Autodesk Inventor part; units mm, degrees
ref_plane "YZ Plane" through (0, 0, 0) normal (1, 0, 0) x (0, 1, 0)
ref_plane "XZ Plane" through (0, 0, 0) normal (0, 1, 0) x (-1, 0, 0)
ref_plane "XY Plane" through (0, 0, 0) normal (0, 0, 1) x (1, 0, 0)
sketch "Sketch1" plane through (0, 0, 0) normal (0, 0, 1) x (1, 0, 0)
  line L0 (-25.4, -38.1) -> (25.4, -38.1) construction
  line L1 (25.4, -38.1) -> (25.4, 38.1) construction
  line L2 (25.4, 38.1) -> (-25.4, 38.1) construction
  line L3 (-25.4, 38.1) -> (-25.4, -38.1) construction
  line L4 (-25.4, -38.1) -> (25.4, 38.1) construction
  line L5 (25.4, -38.1) -> (-25.4, 38.1) construction
  line L6 (25.4, 38.1) -> (-25.4, 38.1) construction
  line L7 (-25.4, 38.1) -> (-25.4, 22.1) construction
  line L8 (-25.4, 22.1) -> (25.4, 22.1) construction
  line L9 (25.4, 22.1) -> (25.4, 38.1) construction
  line L10 (-25.4, -38.1) -> (25.4, -38.1) construction
  line L11 (25.4, -38.1) -> (25.4, -22.1) construction
  line L12 (25.4, -22.1) -> (-25.4, -22.1) construction
  line L13 (-25.4, -22.1) -> (-25.4, -38.1) construction
  line L14 (25.4, -15) -> (-25.4, -15) construction
  line L15 (-25.4, -15) -> (-25.4, 15) construction
  line L16 (-25.4, 15) -> (25.4, 15) construction
  line L17 (25.4, 15) -> (25.4, -15) construction
  line L18 (25.4, -15) -> (-25.4, 15) construction
  line L19 (-25.4, -15) -> (25.4, 15) construction
  line L20 (-25.4, 22.1) -> (-13.4, 22.1) construction
  line L21 (-13.4, 22.1) -> (-13.4, 15) construction
  line L22 (-13.4, 15) -> (-25.4, 15) construction
  line L23 (-25.4, 15) -> (-25.4, 22.1) construction
  line L24 (25.4, -22.1) -> (13.4, -22.1) construction
  line L25 (13.4, -22.1) -> (13.4, -15) construction
  line L26 (13.4, -15) -> (25.4, -15) construction
  line L27 (25.4, -15) -> (25.4, -22.1) construction
  line L28 (-13.4, 15) -> (-6.3, 15) construction
  line L29 (-6.3, 15) -> (-6.3, 22.1) construction
  line L30 (-6.3, 22.1) -> (-13.4, 22.1) construction
  line L31 (-13.4, 22.1) -> (-13.4, 15) construction
  line L32 (13.4, -22.1) -> (6.3, -22.1) construction
  line L33 (6.3, -22.1) -> (6.3, -15) construction
  line L34 (6.3, -15) -> (13.4, -15) construction
  line L35 (13.4, -15) -> (13.4, -22.1) construction
  arc A0 (-9.85, 22.1) -> (-9.85, 15) centre (-9.85, 18.55) ccw construction
  arc A1 (9.85, -22.1) -> (9.85, -15) centre (9.85, -18.55) ccw construction
  line L36 (25.4, 22.1) -> (25.4, 38.1)
  line L37 (25.4, 38.1) -> (-25.4, 38.1)
  line L38 (-25.4, 38.1) -> (-25.4, -15)
  line L39 (-25.4, -15) -> (9.85, -15)
  arc A2 (9.85, -22.1) -> (9.85, -15) centre (9.85, -18.55) ccw
  line L40 (9.85, -22.1) -> (-25.4, -22.1)
  line L41 (-25.4, -22.1) -> (-25.4, -38.1)
  line L42 (-25.4, -38.1) -> (25.4, -38.1)
  line L43 (25.4, -38.1) -> (25.4, 15)
  line L44 (25.4, 15) -> (-9.85, 15)
  arc A3 (-9.85, 22.1) -> (-9.85, 15) centre (-9.85, 18.55) ccw
  line L45 (-9.85, 22.1) -> (25.4, 22.1)
  line L46 (25.4, 38.1) -> (25.4, 22.1)
  line L47 (25.4, 22.1) -> (-9.85, 22.1)
  line L48 (-9.85, 15) -> (25.4, 15)
  line L49 (25.4, 15) -> (25.4, -38.1)
  line L50 (25.4, -38.1) -> (-25.4, -38.1)
  line L51 (-25.4, -38.1) -> (-25.4, -22.1)
  line L52 (-25.4, -22.1) -> (9.85, -22.1)
  line L53 (-25.4, -15) -> (9.85, -15)
  arc A4 (9.85, -22.1) -> (9.85, -15) centre (9.85, -18.55) ccw
  arc A5 (-9.85, 22.1) -> (-9.85, 15) centre (-9.85, 18.55) ccw
  line L54 (-25.4, -15) -> (-25.4, 38.1)
  line L55 (-25.4, 38.1) -> (25.4, 38.1)
  point P0 (0, 0)
  dimension "d0" = 50.8
  dimension "d1" = 76.2
  dimension "d2" = 50.8
  dimension "d3" = 16
  dimension "d4" = 16
  dimension "d5" = 30
  dimension "d6" = 12
  dimension "d7" = 12
  dimension "d8" = 7.1
  dimension "d9" = 7.1
extrude "Extrusion1" add sketch "Sketch1" along normal blind 19
sketch "Sketch2" plane through (-25.4, 38.1, 0) normal (0, 1, 0) x (1, 0, 0)
  line L0 (0, -19) -> (50.8, 0) construction
  line L1 (50.8, -19) -> (0, 0) construction
  point P0 (25.4, 0)
  point P1 (25.4, -9.5)
hole "Hole1" at (0, 38.1, 9.5) direction (0, -1, 0) diameter 10.106 end through all
equation "\"d2\" = d0"
equation "\"d4\" = d3"
properties part number "loadcell_s_500kg" material "Stainless Steel"
The model under review builds one solid part; all positions refer to its coordinate system, in mm. A direction names the side the tool comes from. Round coordinates to 2 decimals unless told otherwise and drop trailing zeros. Write each loop counter-clockwise with the first axis right and the second up, starting at its lowest first coordinate (ties: lowest second). Pieces come first, ordered by that corner, then holes. Notation, with made-up numbers: (-25.75, -13.75) - (5.25, -13.75) arc R16 ccw to (5.25, 12.25) - close; hole circle Ø1 at (62.25, 84). An arc over 180 degrees is marked (long way). One line per item, written item: value. Start each with the question number.
1. Machinability: for faces 4 (the face through (-8, -22.1, 9)), 5 (the face through (8, 15, 9)), 6 (the face through (3.075, -30.212, 5.49)), which of the approach directions +Z, -Z, +X, -X, +Y, -Y give a long, thin tool a straight path to every point of the face, cutting with its end or side? Answer none if there is none.
2. Consider section A-A on x = 0. Write out the cut boundary in (y, z), and give its area (3 significant figures).
3. Consider section C-C on x = 6.5. Write out the cut boundary in (y, z).
4. To check wall thickness, follow L1, parallel to Y at x = -9, z = 10; L2, parallel to X at y = 8, z = 9.5; L3, parallel to Y at x = 16.5, z = 18. State the ranges of each line that lie inside material, in increasing order. Write a range as from..to.
5. Consider section D-D on y = 29. Write out the cut boundary in (x, z), and give its area (3 significant figures).
6. The part is to be moulded in two halves that separate along X. For faces 1 (the face through (-25.4, 12, 9)), 2 (the face through (3.075, 29.988, 5.49)), 3 (the face through (-5.3, 38.1, 9.4)), say which applies: released by +X, released by -X, zero draft, split by the parting line, or undercut.
7. Clearance check with a flat-ended pin moving along its axis: P1, Ø6, axis at x = 0, z = 9.5, coming from the -Y side. State where the tip first meets the part, or that it passes through.
8. Consider section B-B on x = 16. Write out the cut boundary in (y, z).
Checks:
1. face 4: +Z, -Z, -X
1. face 5: +Z, -Z, +X
1. face 6: +Y, -Y
2. outline: (-38.1, 0) - (-22.1, 0) - (-22.1, 4.45) - (-38.1, 4.45) - close; (-38.1, 14.55) - (-22.1, 14.55) - (-22.1, 19) - (-38.1, 19) - close; (-15, 0) - (15, 0) - (15, 4.45) - (-15, 4.45) - close; (-15, 14.55) - (15, 14.55) - (15, 19) - (-15, 19) - close; (22.1, 0) - (38.1, 0) - (38.1, 4.45) - (22.1, 4.45) - close; (22.1, 14.55) - (38.1, 14.55) - (38.1, 19) - (22.1, 19) - close
2. area: 551 mm^2
3. outline: (-38.1, 0) - (-22.1, 0) - (-22.1, 19) - (-38.1, 19) - close; (-15, 0) - (15, 0) - (15, 19) - (-15, 19) - close; (22.1, 0) - (38.1, 0) - (38.1, 19) - (22.1, 19) - close
4. L1: y = -38.1..-22.1, -15..15, 22.1..38.1
4. L2: x = -25.4..-5.05, 5.05..25.4
4. L3: y = -38.1..15, 22.1..38.1
5. outline: (-25.4, 0) - (25.4, 0) - (25.4, 19) - (-25.4, 19) - close; hole circle Ø10.11 at (0, 9.5)
5. area: 885 mm^2
6. face 1: released by -X
6. face 2: undercut
6. face 3: zero draft
7. P1: passes through
8. outline: (-38.1, 0) - (15, 0) - (15, 19) - (-38.1, 19) - close; (22.1, 0) - (38.1, 0) - (38.1, 19) - (22.1, 19) - close
